For this review, take the finished solid that the model builds, in its own axes (mm). A direction names the side the tool comes from. Round coordinates to 2 decimals unless told otherwise and drop trailing zeros. Order: outer loops, then holes, each group sorted by start corner. A loop starts at its lowest first (then second) coordinate and runs counter-clockwise, first axis right, second up. Notation, with made-up numbers: (81.25, 50) -> (118.25, 50) arc R13 cw to (118.25, 56) -> close; hole circle Ø10 at (-6.5, -10). An arc over 180 degrees is marked (long way). Use a Markdown table: item, result. Add a question column.
1) Consider section A-A (y = 0). State the section outline as (x, z) points.
2) Machinability: for faces 1 (the face through (6.35, 0, -2)), 2 (the face through (-1.44, 2.76, 4.19)), which of the approach directions +Z, -Z, +X, -X, +Y, -Y give a long, thin tool a straight path to every point of the face, cutting with its end or side? Answer none if there is none.
3) Wall thickness on line 1 along Z through (x, y) = (-2.5, 1.25); line 2 along Y through (x, z) = (-3.75, -4); line 3 along Y through (x, z) = (1.5, -3.25): over which ranges is each line inside the solid? List them lowest first. Write a range as [from, to].
4) Consider section D-D (z = 4.25). State the section outline as (x, y) points, plus the area to 3 significant figures.
5) Consider section C-C (x = -5). State the section outline as (y, z) points, plus the area to 3 significant figures.
6) Draft analysis for pull direction Z (two halves, no side actions). For faces 3 (the face through (0.52, 2.33, 1.19)), 4 (the face through (-3.131, 5.525, -2.071)), 5 (the face through (0, 0, 6.35)), state which applies: pulls with the +Z half, pulls with the -Z half, needs draft (parallel to the pull), parting line crosses it, or undercut.
7) Clearance check with flat-ended pins moving along their axes: P1, Ø6, axis at x = -2, y = 4, coming from the -Z side; P2, Ø1.5, axis at x = 1, y = -5, coming from the +Z side. State where each tip first meets the part, or that it passes through.
8) Consider section B-B (z = -0.25). State the section outline as (x, y) points.
```python
from build123d import *

# Parameters (mm, degrees)
SKETCH2_OUTSIDE_W  = 33.164
SKETCH2_OUTSIDE_H  = 33.164
CUT_EXTRUDE1_DEPTH = 6.5372
FILLET1_R          = 0.381


with BuildPart() as part:
    # Sketch1 → Revolve1 (revolve)
    with BuildSketch(Plane(origin=(0, 0, 0), x_dir=(0, 0, -1), z_dir=(1, 0, 0)), mode=Mode.PRIVATE) as revolve1_sk:
        with BuildLine():
            Line((0, 11.989122877), (0, 2.3876))
            Line((0, 2.3876), (-1.9812, 2.3876))
            Line((-1.9812, 2.3876), (-2.7051, 3.1115))
            Line((-2.7051, 3.1115), (-5.6261, 3.1115))
            Line((-5.6261, 3.1115), (-6.35, 2.3876))
            Line((-6.35, 2.3876), (-6.35, 0))
            Line((-6.35, 0), (5.5372, 0))
            ThreePointArc((5.5372, 0), (4.086038504, 6.603023005), (0, 11.989122877))
        make_face()
    revolve(revolve1_sk.sketch.rotate(Axis((0, 0, 0), (0, 0, 1)), 90), axis=Axis((0, 0, 0), (0, 0, 1)))  # turned: the seam where the file's is

    # Sketch2 outside → Cut-Extrude1 (cut, through all)
    with BuildSketch(Plane.XY):
        Rectangle(SKETCH2_OUTSIDE_W, SKETCH2_OUTSIDE_H)
        Polygon((0, 7.332348419), (-6.35, 3.666174209), (-6.35, -3.666174209), (0, -7.332348419), (6.35, -3.666174209), (6.35, 3.666174209), align=None, mode=Mode.SUBTRACT)
    extrude(amount=-CUT_EXTRUDE1_DEPTH, mode=Mode.SUBTRACT)

    # Fillet1
    fillet1_edges = [part.edges().sort_by_distance(p)[0] for p in [
        (2.3876, 0, 0),
    ]]
    fillet(fillet1_edges, radius=FILLET1_R)


solid = part.part
```
Results list:
| question | item | result |
|---|---|---|
| 1 | outline | (-6.35, -4.2) arc R15.75 ccw to (6.35, -4.2) -> (6.35, 0) -> (2.77, 0) arc R0.38 cw to (2.39, 0.38) -> (2.39, 1.98) -> (3.11, 2.71) -> (3.11, 5.63) -> (2.39, 6.35) -> (-2.39, 6.35) -> (-3.11, 5.63) -> (-3.11, 2.71) -> (-2.39, 1.98) -> (-2.39, 0.38) arc R0.38 cw to (-2.77, 0) -> (-6.35, 0) -> close |
| 2 | face 1 | +Z, -Z, +X, +Y, -Y |
| 2 | face 2 | +Z |
| 3 | line 1 | [-5.29, 0], [2.39, 5.94] |
| 3 | line 2 | [-5.17, 5.17] |
| 3 | line 3 | [-6.47, 6.47] |
| 4 | outline | circle Ø6.22 at (0, 0) |
| 4 | area | 30.4 mm2 |
| 5 | outline | (-4.45, -4.05) arc R14.93 ccw to (4.45, -4.05) -> (4.45, 0) -> (-4.45, 0) -> close |
| 5 | area | 40.0 mm2 |
| 6 | face 3 | undercut |
| 6 | face 4 | needs draft |
| 6 | face 5 | pulls with the +Z half |
| 7 | P1 | z = -5.47 |
| 7 | P2 | z = 0 |
| 8 | outline | (-6.35, -3.67) -> (0, -7.33) -> (6.35, -3.67) -> (6.35, 3.67) -> (0, 7.33) -> (-6.35, 3.67) -> close |
